from build123d import *

# Parameters (mm, degrees)
CROQUIS1_W              = 69
CROQUIS1_H              = 64.099232263
CROQUIS1_R              = 1
CROQUIS1_R_2            = 1.5
SALIENTE_EXTRUIR1_DEPTH = 2
REDONDEO1_R             = 1


with BuildPart() as part:
    # Croquis1 → Saliente-Extruir1 (new body)
    with BuildSketch(Plane(origin=(0, 0, 0), x_dir=(1, 0, 0), z_dir=(0, 1, 0))):
        with Locations((-35.029110392, 0.70962906)):
            Rectangle(CROQUIS1_W, CROQUIS1_H)
        with BuildLine():
            ThreePointArc((-59.454384172, 4.810651437), (-58.662459069, 5.641041677), (-57.611472837, 5.180475439))
            ThreePointArc((-57.611472837, 5.180475439), (-56.358108465, 0.762709988), (-57.556841461, -3.67019121))
            ThreePointArc((-57.556841461, -3.67019121), (-57.60722938, -3.763799887), (-57.667223738, -3.851562088))
            ThreePointArc((-57.667223738, -3.851562088), (-58.665645829, -4.226208068), (-59.438939328, -3.491889713))
            ThreePointArc((-59.438939328, -3.491889713), (-59.459295474, -3.392138765), (-59.469455013, -3.290840157))
            ThreePointArc((-59.469455013, -3.290840157), (-59.763795222, 0.760467206), (-59.454384172, 4.810651437))
        make_face(mode=Mode.SUBTRACT)
        with Locations((-13.221985845, -5.290370941)):
            Circle(CROQUIS1_R, mode=Mode.SUBTRACT)
        with Locations((-66.45759178, 0.709629059)):
            Circle(CROQUIS1_R_2, mode=Mode.SUBTRACT)
        with Locations((-44.286593268, 0.709629059)):
            Circle(CROQUIS1_R_2, mode=Mode.SUBTRACT)
        with Locations((-25.130085357, 0.709629059)):
            Circle(CROQUIS1_R_2, mode=Mode.SUBTRACT)
        with Locations((-13.221985845, 6.709629059)):
            Circle(CROQUIS1_R, mode=Mode.SUBTRACT)
    extrude(amount=SALIENTE_EXTRUIR1_DEPTH)

    # Redondeo1
    redondeo1_edges = [part.edges().sort_by_distance(p)[0] for p in [
        (-0.529110392, 1, 31.339987072),
        (-69.529110392, 1, 31.339987072),
        (-69.529110392, 1, -32.759245191),
        (-0.529110392, 1, -32.759245191),
    ]]
    fillet(redondeo1_edges, radius=REDONDEO1_R)


solid = part.part
Work out the finished part from the listing and answer in its coordinate system (mm). A direction names the side the tool comes from. Give positions to 0.01 mm unless a question says otherwise; leave off trailing zeros. Order: outer loops, then holes, each group sorted by start corner. A loop starts at its lowest first (then second) coordinate and runs counter-clockwise, first axis right, second up. Notation, with made-up numbers: (85, 10.5) - (132, 10.5) arc R33 ccw to (132, 39.5) - close; hole circle Ø8 at (83, 38). An arc over 180 degrees is marked (long way). Answer as CSV lines item,"result". Start each with the question number.
Q1. Given pin 1 Ø1.2 at (x, z) = (-13.22, -6.71) entering from +Y, flat-ended and moving along its own axis, determine where the tip first touches the part or whether it passes through.
Q2. For faces 4 (the face through (-35, 1, 31.34)), 5 (the face through (-56.36, 0.99, -0.83)), determine the directions among +Z, -Z, +X, -X, +Y, -Y from which every point of the face is accessible in a straight line to the end or side of a thin tool.
Q3. Find the intervals of material crossed by L1, parallel to Z at x = -14, y = 1.1; L2, parallel to X at y = 0.1, z = 0; L3, parallel to X at y = 1.8, z = -1, in increasing order. Write a range as [from, to].
Q4. The mould has two halves that part along X. Classify faces 1 (the face through (-35, 1, -32.759)), 2 (the face through (-69.529, 1, 0)), 3 (the face through (-45.48, 0.99, 0.2)): +X half, -X half, draft (parallel to the pull), parting line (faces both ways), or undercut.
Q5. The part is cut by section A-A (x = -24.5). Write down the section's boundary in (y, z), then the cut area to 3 significant figures.
Check result:
1,pin 1,"passes through"
2,face 4,"+Z, +X, -X, +Y, -Y"
2,face 5,"+Y, -Y"
3,L1,"z = [-32.76, -7.34], [-6.08, 4.66], [5.92, 31.34]"
3,L2,"x = [-69.53, -67.78], [-65.14, -59.75], [-56.39, -45.61], [-42.97, -26.45], [-23.81, -0.53]"
3,L3,"x = [-69.53, -67.93], [-64.99, -59.76], [-56.36, -45.76], [-42.81, -26.6], [-23.66, -0.53]"
4,face 1,"draft"
4,face 2,"-X half"
4,face 3,"undercut"
5,outline,"(0, -32.76) - (2, -32.76) - (2, -2.07) - (0, -2.07) - close; (0, 0.65) - (2, 0.65) - (2, 31.34) - (0, 31.34) - close"
5,area,"123 mm²"
